The drawing under review shows one solid part. Ordinate dimensions are in mm from its lowest x, y, z. A direction names the side the tool comes from. Round coordinates to 2 decimals unless told otherwise and drop trailing zeros. Order: outer loops, then holes, each group sorted by start corner. A loop starts at its lowest first (then second) coordinate and runs counter-clockwise, first axis right, second up.
1) Mouldability with a two-part tool opening along X and no side actions: class the marked faces 4, 5 and 6 as pulls with the +X half, pulls with the -X half, needs draft (parallel to the pull), parting line crosses it, or undercut.
2) Machinability: for the marked faces 1, 2 and 3, which of the approach directions +Z, -Z, +X, -X, +Y, -Y give a long, thin tool a straight path to every point of the face, cutting with its end or side? Answer none if there is none.
3) Consider section C-C (y = 5.5). Give the boundary of the cut face in (x, z), then the cut area to 3 significant figures.
4) Clearance check with flat-ended pins moving along their axes: P1, Ø13.5, axis at x = 39.5, y = 13, coming from the -Z side; P2, Ø6, axis at x = 35, y = 9, coming from the +Z side; P3, Ø2.5, axis at x = 70, z = 95, coming from the +Y side; P4, Ø5, axis at y = 19, z = 38.5, coming from the -X side. State where each tip first meets the part, or that it passes through.
5) Consider section B-B (x = 5). Give the boundary of the cut face in (y, z), then the cut area to 3 significant figures.
6) Consider section A-A (z = 5). Give the boundary of the cut face in (x, y), then the cut area to 3 significant figures.
7) Consider section D-D (z = 30.5). Give the boundary of the cut face in (x, y), then the cut area to 3 significant figures.
8) To check wall thickness, follow L1, parallel to Z at x = 5, y = 31.75; L2, parallel to X at y = 32.75, z = 5; L3, parallel to Z at x = 34, y = 10. State the ranges of each line that lie inside material, in increasing order.
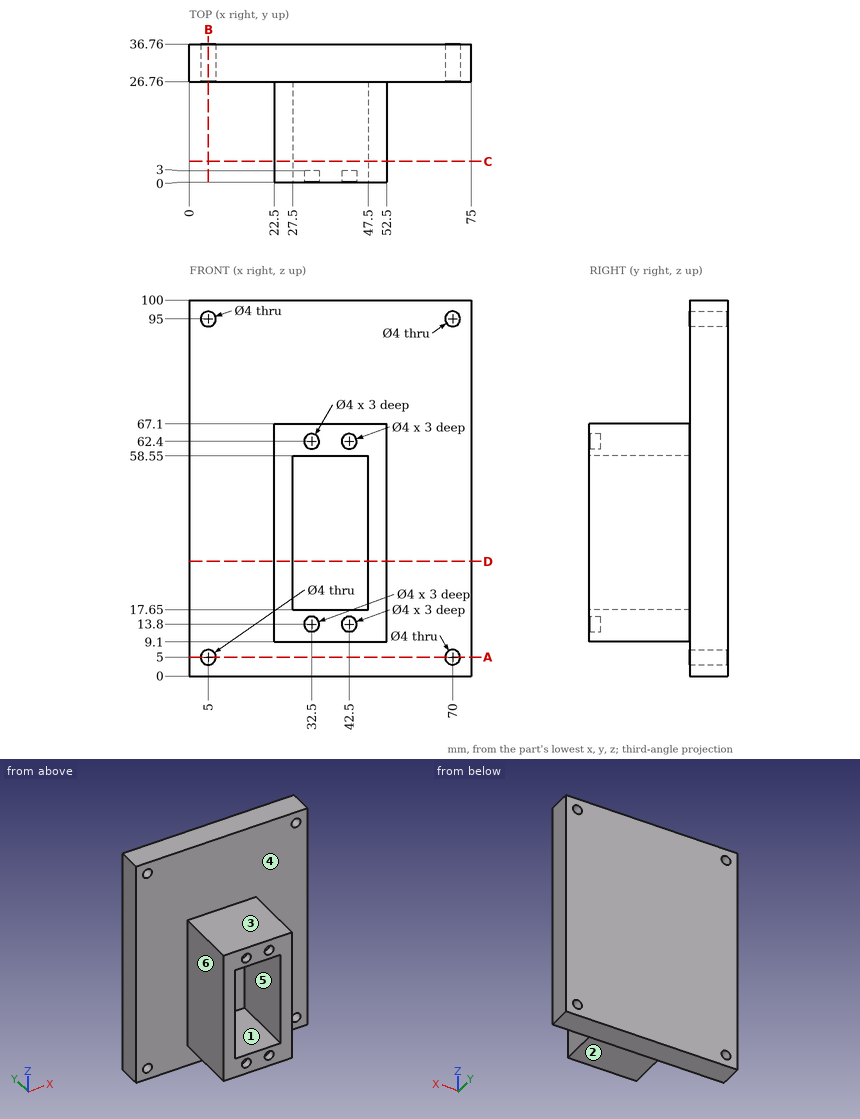
Answer below:
1. face 4: needs draft
1. face 5: undercut
1. face 6: pulls with the -X half
2. face 1: -Y
2. face 2: -Z, +X, -X, -Y
2. face 3: +Z, +X, -X, -Y
3. outline: (22.5, 9.1) - (52.5, 9.1) - (52.5, 67.1) - (22.5, 67.1) - close; hole (27.5, 17.65) - (47.5, 17.65) - (47.5, 58.55) - (27.5, 58.55) - close
3. area: 922 mm2
4. P1: stops at z = 9.1
4. P2: stops at z = 67.1
4. P3: passes through
4. P4: stops at x = 22.5
5. outline: (26.76, 0) - (36.76, 0) - (36.76, 3) - (26.76, 3) - close; (26.76, 7) - (36.76, 7) - (36.76, 93) - (26.76, 93) - close; (26.76, 97) - (36.76, 97) - (36.76, 100) - (26.76, 100) - close
5. area: 920 mm2
6. outline: (0, 26.76) - (3, 26.76) - (3, 36.76) - (0, 36.76) - close; (7, 26.76) - (68, 26.76) - (68, 36.76) - (7, 36.76) - close; (72, 26.76) - (75, 26.76) - (75, 36.76) - (72, 36.76) - close
6. area: 670 mm2
7. outline: (0, 26.76) - (22.5, 26.76) - (22.5, 0) - (27.5, 0) - (27.5, 26.76) - (47.5, 26.76) - (47.5, 0) - (52.5, 0) - (52.5, 26.76) - (75, 26.76) - (75, 36.76) - (0, 36.76) - close
7. area: 1,020 mm2
8. L1: z = 0 to 3, 7 to 93, 97 to 100
8. L2: x = 0 to 3, 7 to 68, 72 to 75
8. L3: z = 9.1 to 17.65, 58.55 to 67.1
